Build history of the part. All positions in model axes, mm. Face numbers are marked on the shaded views. A direction names the side the tool comes from. Round coordinates to 2 decimals unless told otherwise and drop trailing zeros. Write each loop counter-clockwise with the first axis right and the second up, starting at its lowest first coordinate (ties: lowest second). Pieces come first, ordered by that corner, then holes.
1) Wall check: probe 1 along Y at (x, z) = (-157.4, -381.25); probe 2 along X at (y, z) = (45, -399); probe 3 along Z at (x, y) = (-159.25, 43.5). Give the ranges that are in metal, low to high.
2) Saw through at C-C (x = -159.9). Write the cut outline in (y, z).
3) Flat gauge pins, fed straight in: pin 1 (2 mm diameter, centred on y = 42.5, z = -395, fed in from +X); pin 2 (3 mm diameter, centred on x = -160.5, y = 43.5, fed in from -Z); pin 3 (3 mm diameter, centred on y = 43.5, z = -398, fed in from -X). Where does each tip first touch, or does it go through?
4) Pull direction Z, two halves, no side cores. Call the marked faces 1, 2 and 3: +Z half, -Z half, draft (parallel to the pull), parting line (faces both ways), or undercut.
5) Saw through at A-A (z = -381.75). Write the cut outline in (x, y).
6) Saw through at B-B (y = 40.75). Write the cut outline in (x, z).
7) Which spindle directions (+Z, -Z, +X, -X, +Y, -Y) get a long thin tool onto all of the face, cutting with end or side? Do the marked faces 4, 5, 6, 7 and 8. Say none if no direction does.
8) Saw through at D-D (z = -397). Write the cut outline in (x, y).
from build123d import *

# Parameters (mm, degrees)
RESSALTO_EXTRUS_O1_DEPTH = 6
CORTE_EXTRUS_O1_DEPTH    = 389.589061789
ESBO_O3_W                = 1.3
ESBO_O3_H                = 6.5
RESSALTO_EXTRUS_O2_DEPTH = 18
FILETE1_R                = 5
FILETE3_R                = 0.5


with BuildPart() as part:
    # Esboço1 → Ressalto-extrusão1 (new body)
    with BuildSketch(Plane(origin=(-161.802837797, 0, 0), x_dir=(0, 0, -1), z_dir=(1, 0, 0))):
        with BuildLine():
            Line((384.694639655, 46.958533656), (379.194639655, 46.958533656))
            ThreePointArc((379.194639655, 46.958533656), (378.487532874, 46.665640437), (378.194639655, 45.958533656))
            Line((378.194639655, 45.958533656), (378.194639655, 39.458533656))
            ThreePointArc((378.194639655, 39.458533656), (378.487532874, 38.751426875), (379.194639655, 38.458533656))
            Line((379.194639655, 38.458533656), (384.694639655, 38.458533656))
            ThreePointArc((384.694639655, 38.458533656), (385.401746437, 38.751426875), (385.694639655, 39.458533656))
            Line((385.694639655, 39.458533656), (385.694639655, 45.958533656))
            ThreePointArc((385.694639655, 45.958533656), (385.401746437, 46.665640437), (384.694639655, 46.958533656))
        make_face()
    extrude(amount=RESSALTO_EXTRUS_O1_DEPTH)

    # Esboço2 → Corte-extrusão1 (cut, through all)
    with BuildSketch(Plane(origin=(-155.802837797, 0, 0), x_dir=(0, 0, -1), z_dir=(1, 0, 0))):
        with BuildLine():
            Line((380.194639655, 45.958533656), (383.694639655, 45.958533656))
            ThreePointArc((383.694639655, 45.958533656), (384.401746437, 45.665640437), (384.694639655, 44.958533656))
            Line((384.694639655, 44.958533656), (384.694639655, 40.458533656))
            ThreePointArc((384.694639655, 40.458533656), (384.401746437, 39.751426875), (383.694639655, 39.458533656))
            Line((383.694639655, 39.458533656), (380.194639655, 39.458533656))
            ThreePointArc((380.194639655, 39.458533656), (379.487532874, 39.751426875), (379.194639655, 40.458533656))
            Line((379.194639655, 40.458533656), (379.194639655, 44.958533656))
            ThreePointArc((379.194639655, 44.958533656), (379.487532874, 45.665640437), (380.194639655, 45.958533656))
        make_face()
    extrude(amount=-CORTE_EXTRUS_O1_DEPTH, mode=Mode.SUBTRACT)

    # Esboço3 → Ressalto-extrusão2 (add)
    with BuildSketch(Plane(origin=(0, 0, -385.694639655), x_dir=(-1, 0, 0), z_dir=(0, 0, -1))):
        with Locations((158.802837797, 42.708533656)):
            Rectangle(ESBO_O3_W, ESBO_O3_H)
    extrude(amount=RESSALTO_EXTRUS_O2_DEPTH)

    # Filete1
    # the kernel refuses this fillet: 5 mm, written as the material it adds along each edge
    with BuildSketch(Plane(origin=(-159.452837797, 39.458533656, -385.694639655), x_dir=(-1, 0, 0), z_dir=(0, 1, 0)), Plane(origin=(-158.152837797, 45.958533656, -385.694639655), x_dir=(1, 0, 0), z_dir=(0, -1, 0))) as filete1_piece_1:
        with BuildLine():
            CenterArc((5, -4.239988208), FILETE1_R, 122.005454828, 57.994545172)
            Line((0, -4.239988208), (-0.1, -4.239988208))
            Line((-0.1, -4.239988208), (-0.1, 0))
            Line((-0.1, 0), (0, 0.1))
            ThreePointArc((0, 0.1), (1.175, 0.1), (2.297, 0.084799764))
            Line((2.297, 0.084799764), (2.35, 0))
        make_face()
    extrude(amount=6.5)

    # Filete3
    filete3_edges = [part.edges().sort_by_distance(p)[0] for p in [
        (-159.452837797, 42.708533656, -403.694639655),
        (-158.802837797, 45.958533656, -403.694639655),
        (-158.152837797, 42.708533656, -403.694639655),
        (-158.802837797, 39.458533656, -403.694639655),
    ]]
    fillet(filete3_edges, radius=FILETE3_R)


solid = part.part
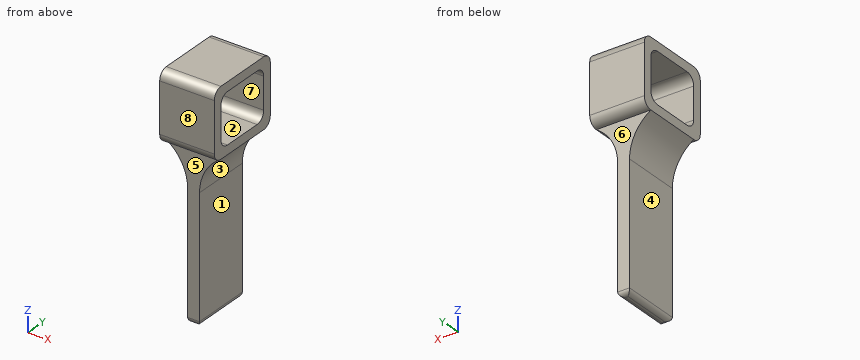
Evaluation:
1. probe 1: y = 38.46 to 39.46, 45.96 to 46.96
1. probe 2: x = -159.45 to -158.15
1. probe 3: z = -403.6 to -384.69, -379.19 to -378.19
2. outline: (38.46, -384.69) arc R1 ccw to (39.46, -385.69) - (39.46, -387.87) - (45.96, -387.87) - (45.96, -385.69) arc R1 ccw to (46.96, -384.69) - (46.96, -379.19) arc R1 ccw to (45.96, -378.19) - (39.46, -378.19) arc R1 ccw to (38.46, -379.19) - close; hole (39.46, -383.69) arc R1 ccw to (40.46, -384.69) - (44.96, -384.69) arc R1 ccw to (45.96, -383.69) - (45.96, -380.19) arc R1 ccw to (44.96, -379.19) - (40.46, -379.19) arc R1 ccw to (39.46, -380.19) - close
3. pin 1: stops at x = -158.15
3. pin 2: stops at z = -403.69
3. pin 3: stops at x = -159.45
4. face 1: draft
4. face 2: undercut
4. face 3: -Z half
5. outline: (-161.8, 38.46) - (-155.8, 38.46) - (-155.8, 39.46) - (-161.8, 39.46) - close; (-161.8, 45.96) - (-155.8, 45.96) - (-155.8, 46.96) - (-161.8, 46.96) - close
6. outline: (-161.8, -385.69) arc R5 cw to (-159.45, -389.93) - (-159.45, -403.19) arc R0.5 ccw to (-158.95, -403.69) - (-158.65, -403.69) arc R0.5 ccw to (-158.15, -403.19) - (-158.15, -389.93) arc R5 cw to (-155.8, -385.69) - (-155.8, -384.69) - (-161.8, -384.69) - close; (-161.8, -379.19) - (-155.8, -379.19) - (-155.8, -378.19) - (-161.8, -378.19) - close
7. face 4: -Z, -X, +Y, -Y
7. face 5: -Z, +X, -X, -Y
7. face 6: -Z, +X, -X, +Y
7. face 7: +X, -X
7. face 8: +Z, -Z, +X, -X, -Y
8. outline: (-159.45, 39.46) - (-158.15, 39.46) - (-158.15, 45.96) - (-159.45, 45.96) - close
